Work out the finished part from the listing and answer in its coordinate system (mm). A direction names the side the tool comes from. Give positions to 0.01 mm unless a question says otherwise; leave off trailing zeros. Loops run counter-clockwise (first coordinate to the right, second up) from the corner with the lowest first, then second, coordinate; pieces in that order, holes last. Notation, with made-up numbers: (-17, 80) -> (26, 80) arc R27 cw to (26, 109) -> close; hole circle Ø1 at (73.25, 40). An arc over 180 degrees is marked (long way). Answer as CSV lines item,"result". Start each with the question number.
1. Find the intervals of material crossed by line 1 along X through (y, z) = (-5, 0); line 2 along Y through (x, z) = (2.5, 8.5); line 3 along Z through (x, y) = (-6.5, -16), in increasing order.
2. Find section C-C, the plane y = -13.5. Give the vertices of the cut face in (x, z).
3. A tool of negligible diameter and unlimited length cuts with its end or side. For faces 4 (the face through (-8, -12, 12.5)), 5 (the face through (10.4, -22.5, 0.9)), 6 (the face through (-12, -27, -7.5)), from which of +Z, -Z, +X, -X, +Y, -Y can it reach the whole face along a straight path? Write none if from no direction.
4. Find section A-A, the plane z = 0. Give the vertices of the cut face in (x, y), and give its area (3 significant figures).
5. Flat-ended cylindrical pins translate along their axes: pin 1 Ø10 at (y, z) = (-21, 13.5) entering from +X; pin 2 Ø12.5 at (x, z) = (-10, 1.5) entering from -Y; pin 3 Ø11 at (x, y) = (-10.5, -15) entering from -Z; pin 4 Ø3 at (x, y) = (-2, -15) entering from +Z. Find the tip coordinate at first contact, or state that the pin passes through.
6. Determine the mould class of faces 1 (the face through (-11, -17.5, -10)), 2 (the face through (-3.36, -24.96, 9.55)), 3 (the face through (19.524, -16.05, -4.336)) for opening direction X: +X half, -X half, draft (parallel to the pull), parting line (faces both ways), or undercut.
7. Find section B-B, the plane y = -5. Give the vertices of the cut face in (x, z).
from build123d import *

# Parameters (mm, degrees)
SKETCH1_R           = 20
BOSS_EXTRUDE1_DEPTH = 7.5
SKETCH2_R           = 20
SKETCH2_R_2         = 12.5
BOSS_EXTRUDE2_DEPTH = 15
SKETCH3_R           = 20
BOSS_EXTRUDE3_DEPTH = 10
CUT_EXTRUDE2_DEPTH  = 5
CUT_EXTRUDE3_DEPTH  = 44.084219849
SKETCH6_R           = 8
CUT_EXTRUDE4_DEPTH  = 5
SKETCH7_R           = 2.1
CUT_EXTRUDE5_DEPTH  = 4.5
SKETCH8_R           = 1
CUT_EXTRUDE6_DEPTH  = 41.868692174
FILLET1_R           = 1.5
FILLET2_R           = 2


with BuildPart() as part:
    # Sketch1 → Boss-Extrude1 (new body)
    with BuildSketch(Plane(origin=(0, 0, 0), x_dir=(1, 0, 0), z_dir=(0, 1, 0))):
        with Locations(Location((0, 0, 0), (0, 0, 270))):
            Circle(SKETCH1_R)
    extrude(amount=-BOSS_EXTRUDE1_DEPTH)

    # Sketch2 → Boss-Extrude2 (add)
    with BuildSketch(Plane.XZ.offset(7.5)):
        with Locations(Location((0, 0, 0), (0, 0, 90))):
            Circle(SKETCH2_R)
        with Locations(Location((0, 0, 0), (0, 0, 270))):
            Circle(SKETCH2_R_2, mode=Mode.SUBTRACT)
    extrude(amount=BOSS_EXTRUDE2_DEPTH)

    # Sketch3 → Boss-Extrude3 (add)
    with BuildSketch(Plane.XZ.offset(22.5)):
        with Locations(Location((0, 0, 0), (0, 0, 90))):
            Circle(SKETCH3_R)
    extrude(amount=BOSS_EXTRUDE3_DEPTH)

    # Sketch4 → Cut-Extrude2 (cut)
    with BuildSketch(Plane(origin=(0, -22.5, 0), x_dir=(-1, 0, 0), z_dir=(0, -1, 0))):
        Polygon((10.164510853, 5.47869076), (0.337570049, 11.542069996), (-9.826940805, 6.063379236), (-10.164510853, -5.47869076), (-0.337570049, -11.542069996), (9.826940805, -6.063379236), align=None)
    extrude(amount=CUT_EXTRUDE2_DEPTH, mode=Mode.SUBTRACT)

    # Sketch5 → Cut-Extrude3 (cut, through all)
    with BuildSketch(Plane(origin=(0, 0, 0), x_dir=(0, 0, -1), z_dir=(1, 0, 0))):
        Polygon((7.5, -17.5), (12.5, -17.5), (12.5, -7.5), (-12.5, -7.5), (-12.5, -17.5), (-7.5, -17.5), (-7.5, -32.5), (7.5, -32.5), align=None)
    extrude(amount=-CUT_EXTRUDE3_DEPTH, mode=Mode.SUBTRACT)

    # Sketch6 → Cut-Extrude4 (cut)
    with BuildSketch(Plane.XZ.offset(32.5)):
        Circle(SKETCH6_R)
    extrude(amount=-CUT_EXTRUDE4_DEPTH, mode=Mode.SUBTRACT)

    # Sketch7 → Cut-Extrude5 (cut)
    with BuildSketch(Plane.XZ.offset(7.5)):
        with Locations(Location((0, 0, 0), (0, 0, 270))):
            Circle(SKETCH7_R)
    extrude(amount=-CUT_EXTRUDE5_DEPTH, mode=Mode.SUBTRACT)

    # Sketch8 → Cut-Extrude6 (cut, through all)
    with BuildSketch(Plane.XZ.offset(3)):
        with Locations(Location((0, 0, 0), (0, 0, 270))):
            Circle(SKETCH8_R)
    extrude(amount=-CUT_EXTRUDE6_DEPTH, mode=Mode.SUBTRACT)

    # Fillet1
    fillet1_edges = [part.edges().sort_by_distance(p)[0] for p in [
        (0, -7.5, 2.1),
    ]]
    fillet(fillet1_edges, radius=FILLET1_R)

    # Fillet2
    fillet2_edges = [part.edges().sort_by_distance(p)[0] for p in [
        (0, 0, -20),
        (16.583123952, -32.5, -11.180339887),
    ]]
    fillet(fillet2_edges, radius=FILLET2_R)


solid = part.part
Resolved:
1,line 1,"x = -20 to -2.1, 2.1 to 20"
1,line 2,"y = -32.5 to -27.5, -7.5 to 0"
1,line 3,"z = -18.91 to -12.5, 12.5 to 18.91"
2,outline,"(-15.61, -12.5) arc R20 ccw (long way) to (-15.61, 12.5) -> (0, 12.5) arc R12.5 cw to (0, -12.5) -> close"
3,face 4,"-X"
3,face 5,"none"
3,face 6,"-X, -Y"
4,outline,"(-20, -7.5) -> (-3.6, -7.5) arc R1.5 ccw to (-2.1, -6) -> (-2.1, -3) -> (-1, -3) -> (-1, 0) -> (-18, 0) arc R2 ccw to (-20, -2) -> close; (1, -3) -> (2.1, -3) -> (2.1, -6) arc R1.5 ccw to (3.6, -7.5) -> (12.5, -7.5) -> (12.5, -22.5) -> (10, -22.5) -> (10, -27.5) -> (8, -27.5) -> (8, -32.5) -> (18, -32.5) arc R2 ccw to (20, -30.5) -> (20, -2) arc R2 ccw to (18, 0) -> (1, 0) -> close"
4,area,"494 mm^2"
5,pin 1,"stops at x = 18.1"
5,pin 2,"stops at y = -32.5"
5,pin 3,"stops at z = -19.36"
5,pin 4,"stops at z = 19.99"
6,face 1,"draft"
6,face 2,"undercut"
6,face 3,"parting line"
7,outline,"circle Ø40 at (0, 0); hole circle Ø4.2 at (0, 0)"
